Geometry check sheet. Reference: the model listing, model coordinates, mm. A direction names the side the tool comes from. Coordinates: 2 decimals unless noted, no trailing zeros. Write each loop counter-clockwise with the first axis right and the second up, starting at its lowest first coordinate (ties: lowest second). Pieces come first, ordered by that corner, then holes.
from build123d import *

# Parameters (mm, degrees)
SKETCH1_W           = 40
SKETCH1_H           = 70
SKETCH1_R           = 7.5
BOSS_EXTRUDE1_DEPTH = 30
CUT_EXTRUDE1_DEPTH  = 20
SKETCH3_W           = 40
SKETCH3_H           = 50
CUT_EXTRUDE2_DEPTH  = 15
FILLET1_R           = 15


with BuildPart() as part:
    # Sketch1 → Boss-Extrude1 (new body)
    with BuildSketch(Plane.XY):
        with Locations((0, 15)):
            Rectangle(SKETCH1_W, SKETCH1_H)
        Circle(SKETCH1_R, mode=Mode.SUBTRACT)
    extrude(amount=BOSS_EXTRUDE1_DEPTH)

    # Sketch2 → Cut-Extrude1 (cut)
    with BuildSketch(Plane(origin=(0, 50, 0), x_dir=(1, 0, 0), z_dir=(0, 1, 0))):
        with BuildLine():
            ThreePointArc((7.5, -15), (2.371708245, -7.884875265), (-6, -10.5))
            Line((-6, -10.5), (6, -19.5))
            ThreePointArc((6, -19.5), (7.115124735, -17.371708245), (7.5, -15))
        make_face()
        with BuildLine():
            Line((6, -19.5), (-6, -10.5))
            ThreePointArc((-6, -10.5), (-4.5, -21), (6, -19.5))
        make_face()
    extrude(amount=-CUT_EXTRUDE1_DEPTH, mode=Mode.SUBTRACT)

    # Sketch3 → Cut-Extrude2 (cut)
    with BuildSketch(Plane.XY.offset(30)):
        with Locations((0, 5)):
            Rectangle(SKETCH3_W, SKETCH3_H)
    extrude(amount=-CUT_EXTRUDE2_DEPTH, mode=Mode.SUBTRACT)

    # Fillet1
    # the kernel refuses this fillet: 15 mm, written as the material it takes off along each edge
    with BuildSketch(Plane(origin=(20, -20, -37.5), x_dir=(0, 1, 0), z_dir=(0, 0, 1))) as fillet1_piece_1:
        with BuildLine():
            CenterArc((FILLET1_R, FILLET1_R), FILLET1_R, 180, 90)
            Line((0, FILLET1_R), (0, 0))
            Line((0, 0), (FILLET1_R, 0))
        make_face()
    extrude(amount=90, mode=Mode.SUBTRACT)
    with BuildSketch(Plane(origin=(-20, -20, -37.5), x_dir=(0, 1, 0), z_dir=(0, 0, 1))) as fillet1_piece_2:
        with BuildLine():
            CenterArc((FILLET1_R, -FILLET1_R), FILLET1_R, 90, 90)
            Line((0, -FILLET1_R), (0, 0))
            Line((0, 0), (FILLET1_R, 0))
        make_face()
    extrude(amount=90, mode=Mode.SUBTRACT)
    with BuildSketch(Plane(origin=(-20, 30, 67.5), x_dir=(0, 1, 0), z_dir=(0, 0, -1))) as fillet1_piece_3:
        with BuildLine():
            CenterArc((FILLET1_R, FILLET1_R), FILLET1_R, 180, 90)
            Line((0, FILLET1_R), (0, 0))
            Line((0, 0), (FILLET1_R, 0))
        make_face()
    extrude(amount=52.5, mode=Mode.SUBTRACT)
    with BuildSketch(Plane(origin=(20, 30, 67.5), x_dir=(0, 1, 0), z_dir=(0, 0, -1))) as fillet1_piece_4:
        with BuildLine():
            CenterArc((FILLET1_R, -FILLET1_R), FILLET1_R, 90, 90)
            Line((0, -FILLET1_R), (0, 0))
            Line((0, 0), (FILLET1_R, 0))
        make_face()
    extrude(amount=52.5, mode=Mode.SUBTRACT)


solid = part.part
1. Sectioned sample at C-C, the plane z = 5.5. Record the boundary of the cut face in (x, y), and give its area (3 significant figures).
Computed values:
outline: (-20, -5) arc R15 ccw to (-5, -20) - (5, -20) arc R15 ccw to (20, -5) - (20, 50) - (-20, 50) - close; hole circle Ø15 at (0, 0)
area: 2,530 mm2
2. Sectioned sample at B-B, the plane y = 0. Record the boundary of the cut face in (x, z).
Computed values:
outline: (-20, 0) - (-7.5, 0) - (-7.5, 15) - (-20, 15) - close; (7.5, 0) - (20, 0) - (20, 15) - (7.5, 15) - close
3. Draft check along X on faces 1 (the flat face through (0, 15, 0)), 2 (the flat face through (0, 30, 12)), 3 (the cylindrical face through (-15.49, 34.28, 22.61)). Enter one of: released by +X, released by -X, zero draft, split by the parting line, or undercut.
Computed values:
face 1: zero draft
face 2: undercut
face 3: released by -X
4. Sectioned sample at A-A, the plane x = 0. Record the boundary of the cut face in (y, z), and give its area (3 significant figures).
Computed values:
outline: (-20, 0) - (-7.5, 0) - (-7.5, 15) - (-20, 15) - close; (7.5, 0) - (50, 0) - (50, 7.5) - (30, 7.5) - (30, 15) - (7.5, 15) - close; (30, 22.5) - (50, 22.5) - (50, 30) - (30, 30) - close
area: 825 mm2
5. Sectioned sample at D-D, the plane y = 35. Record the boundary of the cut face in (x, z).
Computed values:
outline: (-20, 0) - (20, 0) - (20, 15) - (16.18, 15) - (16.18, 30) - (-16.18, 30) - (-16.18, 15) - (-20, 15) - close; hole circle Ø15 at (0, 15)
6. Access from +Z, -Z, +X, -X, +Y, -Y to the whole of each face (thin tool, end or side, straight path). Record for faces 4 (the flat face through (0, 30, 26)), 5 (the cylindrical face through (15.72, 34.51, 22.61)), 6 (the flat face through (-20, 22, 8)).
Computed values:
face 4: +Z, +X, -X, -Y
face 5: +Z, +X, -Y
face 6: +Z, -Z, -X, +Y, -Y
7. Thickness scan on line 1 along Y through (x, z) = (0, 11.25); line 2 along X through (y, z) = (0, 4); line 3 along Z through (x, y) = (-13, 11). Record the ranges inside material, lowest first.
Computed values:
line 1: y = -20 to -7.5, 7.5 to 30
line 2: x = -20 to -7.5, 7.5 to 20
line 3: z = 0 to 15
8. Gauge pin test, flat ends, axial feed: pin 1 Ø2 at (x, z) = (-2, 12) entering from +Y; pin 2 Ø12 at (x, y) = (10.5, 27.5) entering from +Z; pin 3 Ø19.5 at (x, y) = (0, 0) entering from +Z; pin 4 Ø8 at (x, z) = (-13.5, 7.5) entering from -Y. Record the tip position at first contact, or that the pin passes through.
Computed values:
pin 1: stops at y = 30
pin 2: stops at z = 30
pin 3: stops at z = 15
pin 4: stops at y = -19.31
